Input: dimensioned drawing with shaded views. Units: mm. Origin: part minimum x, y, z. A direction names the side the tool comes from. Give positions to 0.01 mm unless a question says otherwise; leave off trailing zeros. Write each loop counter-clockwise with the first axis right and the second up, starting at its lowest first coordinate (ties: lowest second). Pieces come first, ordered by that corner, then holes.
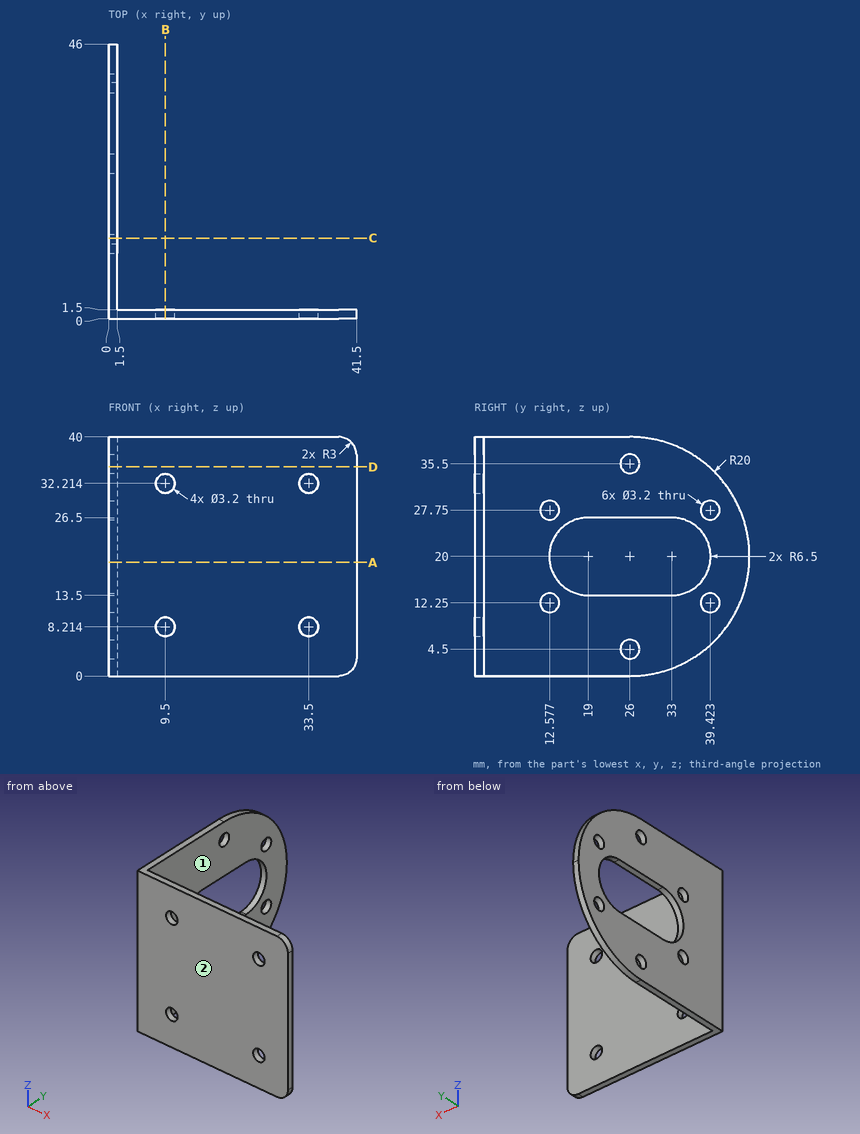
1. Cut plane A-A, the plane z = 19. Return the cut outline in (x, y) (1 decimal).
2. Access query for the marked faces 1 and 2. Directions: +Z, -Z, +X, -X, +Y, -Y. A direction counts if a zero-diameter tool reaches every point of the face in a straight line with its end or side. Return the directions, or none.
3. Cut plane D-D, the plane z = 35. Return the cut outline in (x, y), then the cut area to 3 significant figures.
4. Line query: L1, parallel to Z at x = 9.5, y = 0.5; L2, parallel to Y at x = 1.15, z = 12.25; L3, parallel to Y at x = 34, z = 6. Output: solid intervals per line, ascending.
5. Contact query for flat-ended pins moving along their axis: P1, Ø3.5, axis at y = 12.58, z = 27.75, coming from the -X side; P2, Ø8, axis at x = 26.5, z = 35.5, coming from the +Y side; P3, Ø4, axis at y = 12.58, z = 12.25, coming from the +X side. Output: stop coordinate, or through.
6. Cut plane B-B, the plane x = 9.5. Return the cut outline in (y, z).
7. Cut plane C-C, the plane y = 13.5. Return the cut outline in (x, z).
Response values:
1. outline: (0, 0) - (41.5, 0) - (41.5, 1.5) - (1.5, 1.5) - (1.5, 12.6) - (0, 12.6) - close; (0, 39.4) - (1.5, 39.4) - (1.5, 46) - (0, 46) - close
2. face 1: +Z, -Z, +X, +Y
2. face 2: +Z, -Z, +X, -X, -Y
3. outline: (0, 0) - (41.5, 0) - (41.5, 1.5) - (1.5, 1.5) - (1.5, 24.48) - (0, 24.48) - close; (0, 27.52) - (1.5, 27.52) - (1.5, 39.23) - (0, 39.23) - close
3. area: 114 mm2
4. L1: z = 0 to 6.61, 9.81 to 30.61, 33.81 to 40
4. L2: y = 0 to 10.98, 14.18 to 37.82, 41.02 to 44.44
4. L3: y = 0 to 1.5
5. P1: stops at x = 0
5. P2: stops at y = 1.5
5. P3: stops at x = 1.5
6. outline: (0, 0) - (1.5, 0) - (1.5, 6.61) - (0, 6.61) - close; (0, 9.81) - (1.5, 9.81) - (1.5, 30.61) - (0, 30.61) - close; (0, 33.81) - (1.5, 33.81) - (1.5, 40) - (0, 40) - close
7. outline: (0, 0) - (1.5, 0) - (1.5, 10.94) - (0, 10.94) - close; (0, 13.56) - (1.5, 13.56) - (1.5, 16.54) - (0, 16.54) - close; (0, 23.46) - (1.5, 23.46) - (1.5, 26.44) - (0, 26.44) - close; (0, 29.06) - (1.5, 29.06) - (1.5, 40) - (0, 40) - close
